For this review, take the finished solid that the model builds, in its own axes (mm). A direction names the side the tool comes from. Give positions to 0.01 mm unless a question says otherwise; leave off trailing zeros. Write each loop counter-clockwise with the first axis right and the second up, starting at its lowest first coordinate (ties: lowest second). Pieces come first, ordered by that corner, then holes.
Q1. Mouldability with a two-part tool opening along Y and no side actions: class faces 1 (the flat face through (0, -1, 3)), 2 (the flat face through (5, -2, 0)), 3 (the flat face through (6.99, 0.38, 3.96)) as released by +Y, released by -Y, zero draft, split by the parting line, or undercut.
Q2. We need section A-A (x = 0). Write out the cut boundary in (y, z).
Q3. Machinability: for faces 4 (the flat face through (4.487, 0.365, 1.479)), 5 (the cylindrical face through (6.68, 0.71, 7.7)), which of the approach directions +Z, -Z, +X, -X, +Y, -Y give a long, thin tool a straight path to every point of the face, cutting with its end or side? Answer none if there is none.
Q4. For line 1 (Y direction, x = 0, z = 6); line 2 (Y direction, x = -0.5, z = 1); line 3 (Y direction, x = 0.25, z = 5.5), list the stretches that pass through material, from the lowest coordinate up.
Q5. Insertion check: P1, Ø2, axis at x = 2.5, z = 2.5, coming from the +Y side; P2, Ø1, axis at y = -11, z = 2, coming from the -X side. Each pin has a flat end and moves straight along its axis. Give the tip position at first contact, or say it passes through.
Q6. We need section B-B (z = 7.5). Write out the cut boundary in (x, y), then the cut area to 3 significant figures.
```python
from build123d import *

# Parameters (mm, degrees)
PAD_DEPTH       = 8
SKETCH001_R     = 1
POCKET_DEPTH    = 8.001
POCKET001_DEPTH = 3
FILLET_R        = 1
FILLET001_R     = 1


with BuildPart() as part:
    # Sketch → Pad (new body)
    with BuildSketch(Plane.XY):
        with BuildLine():
            ThreePointArc((5.980892, 13.018408), (0, 18.539936), (-5.980892, 13.018408))
            Line((-5.980892, 13.018408), (-7.974522, -11.901974))
            ThreePointArc((-7.974522, -11.901974), (0, -20.539936), (7.974522, -11.901974))
            Line((7.974522, -11.901974), (5.980892, 13.018408))
        make_face()
    extrude(amount=PAD_DEPTH)

    # Sketch001 (on Face6 of Pad) → Pocket (cut, through all)
    with BuildSketch(Plane.XY.offset(8)):
        with Locations((0, 16.24)):
            Circle(SKETCH001_R)
        with Locations((0.127267, -18)):
            Circle(SKETCH001_R)
    extrude(amount=-POCKET_DEPTH, mode=Mode.SUBTRACT)

    # Sketch002 (on Face4 of Pocket) → Pocket001 (cut)
    with BuildSketch(Plane(origin=(0, 0, 0), x_dir=(1, 0, 0), z_dir=(0, 0, -1))):
        with BuildLine():
            ThreePointArc((4.993762, 9.762804), (0, 15.012492), (-4.993762, 9.762804))
            Line((-4.993762, 9.762804), (-3.995009, -10.212243))
            ThreePointArc((-3.995009, -10.212243), (0, -14.012492), (3.995009, -10.212243))
            Line((3.995009, -10.212243), (4.993762, 9.762804))
        make_face()
    extrude(amount=-POCKET001_DEPTH, mode=Mode.SUBTRACT)

    # Fillet
    fillet_edges = [part.edges().sort_by_distance(p)[0] for p in [
        (-6.977707, 0.558217, 8),
    ]]
    fillet(fillet_edges, radius=FILLET_R)

    # Fillet001
    fillet001_edges = [part.edges().sort_by_distance(p)[0] for p in [
        (-6.977707, 0.558217, 0),
    ]]
    fillet(fillet001_edges, radius=FILLET001_R)


solid = part.part
```
Computed:
1. face 1: undercut
1. face 2: zero draft
1. face 3: released by +Y
2. outline: (-20.54, 1) arc R1 ccw to (-19.54, 0) - (-18.99, 0) - (-18.99, 8) - (-19.54, 8) arc R1 ccw to (-20.54, 7) - close; (-17.01, 0) - (-15.01, 0) - (-15.01, 3) - (14.01, 3) - (14.01, 0) - (15.24, 0) - (15.24, 8) - (-17.01, 8) - close; (17.24, 0) - (17.54, 0) arc R1 ccw to (18.54, 1) - (18.54, 7) arc R1 ccw to (17.54, 8) - (17.24, 8) - close
3. face 4: -Z
3. face 5: +Z, +X, +Y
4. line 1: y = -20.54 to -18.99, -17.01 to 15.24, 17.24 to 18.54
4. line 2: y = -20.52 to -18.78, -17.22 to -14.99, 13.98 to 15.37, 17.11 to 18.52
4. line 3: y = -20.54 to -18.99, -17.01 to 15.27, 17.21 to 18.53
5. P1: stops at y = 18.35
5. P2: stops at x = -7.94
6. outline: (-7.84, -11.91) arc R7.87 ccw (long way) to (7.84, -11.91) - (5.85, 13.01) arc R5.87 ccw to (-5.85, 13.01) - close; hole circle Ø2 at (0, 16.24); hole circle Ø2 at (0.13, -18)
6. area: 490 mm2
